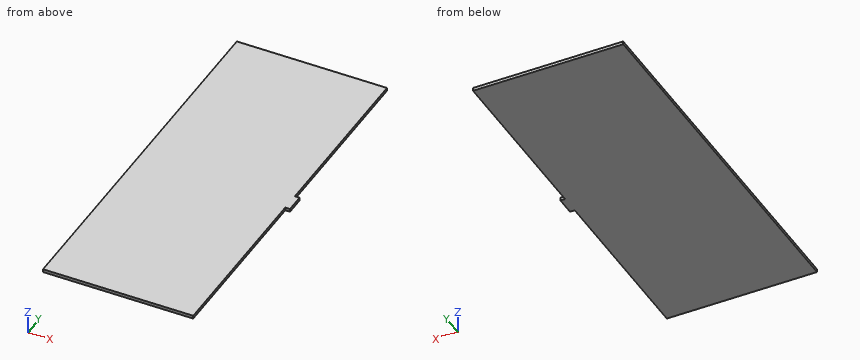
```python
from build123d import *

# Parameters (mm, degrees)
F0_W     = 117.65
F0_H     = 2
F0_W_2   = 12
F1_DEPTH = 96
F2_DEPTH = 3
F3_DEPTH = 2
F4_DEPTH = 2
F5_DEPTH = 1
F6_DEPTH = 1


with BuildPart() as f1:
    # F0 (on Right) → F1 (new body)
    with BuildSketch(Plane.YZ):
        with Locations((244.2264966011, 75.535411799)):
            Rectangle(F0_W, F0_H)
        with Locations((179.4014966011, 75.535411799)):
            Rectangle(F0_W_2, F0_H)
        with Locations((114.5764966011, 75.535411799)):
            Rectangle(F0_W, F0_H)
    extrude(amount=-F1_DEPTH)

    # F0 (on Right) → F2 (join)
    with BuildSketch(Plane.YZ):
        with Locations((179.4014966011, 75.535411799)):
            Rectangle(F0_W_2, F0_H)
    extrude(amount=F2_DEPTH)

    # F3 (cut): a face of the model
    f3_faces = [f1.faces().sort_by_distance(p)[0] for p in [
        (-48, 55.7514966011, 75.535411799),
    ]]
    extrude(f3_faces, amount=-F3_DEPTH, mode=Mode.SUBTRACT)

    # F4 (cut): a face of the model
    f4_faces = [f1.faces().sort_by_distance(p)[0] for p in [
        (-48, 303.0514966011, 75.535411799),
    ]]
    extrude(f4_faces, amount=-F4_DEPTH, mode=Mode.SUBTRACT)

    # F5 (cut): a face of the model
    f5_faces = [f1.faces().sort_by_distance(p)[0] for p in [
        (-48, 57.7514966011, 75.535411799),
    ]]
    extrude(f5_faces, amount=-F5_DEPTH, mode=Mode.SUBTRACT)

    # F6 (cut): a face of the model
    f6_faces = [f1.faces().sort_by_distance(p)[0] for p in [
        (-48, 301.0514966011, 75.535411799),
    ]]
    extrude(f6_faces, amount=-F6_DEPTH, mode=Mode.SUBTRACT)


solid = f1.part
```
Input: part model. Units: mm. Frame: model coordinates. Coordinates: 2 decimals unless noted, no trailing zeros. Loops run counter-clockwise (first coordinate to the right, second up) from the corner with the lowest first, then second, coordinate; pieces in that order, holes last. Notation, with made-up numbers: M 81,19.5 L 114,19.5 A25 ccw 114,57.5 Z; hole C 59,17.25 d4. An arc over 180 degrees is marked long. Use a Markdown table: item, result. Add a question column.
1) Section A-A, the plane z = 74.95. Return the cut outline in (x, y), plus the area to 3 significant figures.
2) Section B-B, the plane y = 263. Return the cut outline in (x, z).
3) Pin query (flat end, axial travel): P1, Ø1, axis at x = 1, z = 75.5, coming from the -Y side; P2, Ø1, axis at y = 140, z = 75.5, coming from the +X side. Return the tip coordinate at first contact, or that it passes through.
4) Line query: L1, parallel to X at y = 211.5, z = 75.65. Output: solid intervals per line, ascending. Write a range as from..to.
Answer below:
| question | item | result |
|---|---|---|
| 1 | outline | M -96,58.75 L 0,58.75 L 0,173.4 L 3,173.4 L 3,185.4 L 0,185.4 L 0,300.05 L -96,300.05 Z |
| 1 | area | 23,200 mm2 |
| 2 | outline | M -96,74.54 L 0,74.54 L 0,76.54 L -96,76.54 Z |
| 3 | P1 | y = 173.4 |
| 3 | P2 | x = 0 |
| 4 | L1 | -96..0 |
